from build123d import *

# Parameters (mm, degrees)
SKETCH1_W           = 38.1
SKETCH1_H           = 25.4
BOSS_EXTRUDE1_DEPTH = 90.1598
SKETCH2_W           = 25.4
SKETCH2_H           = 40.96
BOSS_EXTRUDE2_DEPTH = 30.0228
SKETCH3_W           = 25.4
SKETCH3_H           = 40.96
BOSS_EXTRUDE3_DEPTH = 30.0228
BOSS_EXTRUDE4_DEPTH = 110.0074
BOSS_EXTRUDE5_DEPTH = 110.0074
SKETCH8_R           = 3.81
CUT_EXTRUDE1_DEPTH  = 25.4


with BuildPart() as part:
    # Sketch1 → Boss-Extrude1 (new body)
    with BuildSketch(Plane(origin=(0, 0, 0), x_dir=(1, 0, 0), z_dir=(0, 1, 0))):
        with Locations((5.061883246, 0.142486096)):
            Rectangle(SKETCH1_W, SKETCH1_H)
    extrude(amount=BOSS_EXTRUDE1_DEPTH)

    # Sketch2 → Boss-Extrude2 (add)
    with BuildSketch(Plane(origin=(24.111883246, 0, 0), x_dir=(0, 0, -1), z_dir=(1, 0, 0))):
        with Locations((0.142486096, 69.6798)):
            Rectangle(SKETCH2_W, SKETCH2_H)
    extrude(amount=BOSS_EXTRUDE2_DEPTH)

    # Sketch3 → Boss-Extrude3 (add)
    with BuildSketch(Plane.ZY.offset(13.988116754)):
        with Locations((-0.142486096, 69.6798)):
            Rectangle(SKETCH3_W, SKETCH3_H)
    extrude(amount=BOSS_EXTRUDE3_DEPTH)

    # Sketch4 → Boss-Extrude4 (add)
    with BuildSketch(Plane(origin=(0, 0, -12.842486096), x_dir=(-1, 0, 0), z_dir=(0, 0, -1))):
        Polygon((-54.134683246, 90.1598), (-54.134683246, 49.1998), (-34.576683246, 49.1998), (-34.576683246, 70.6018), align=None)
    extrude(amount=BOSS_EXTRUDE4_DEPTH)

    # Sketch5 → Boss-Extrude5 (add)
    with BuildSketch(Plane(origin=(0, 0, -12.842486096), x_dir=(-1, 0, 0), z_dir=(0, 0, -1))):
        Polygon((44.010916754, 90.1598), (44.010916754, 49.1998), (24.452916754, 49.1998), (24.452916754, 70.6018), align=None)
    extrude(amount=BOSS_EXTRUDE5_DEPTH)

    # Sketch8 → Cut-Extrude1 (cut)
    with BuildSketch(Plane.XZ):
        with Locations(Location((-4.938116754, -0.142486096, 0), (0, 0, 270))):
            Circle(SKETCH8_R)
        with Locations(Location((15.061883246, -0.142486096, 0), (0, 0, 270))):
            Circle(SKETCH8_R)
    extrude(amount=-CUT_EXTRUDE1_DEPTH, mode=Mode.SUBTRACT)


solid = part.part
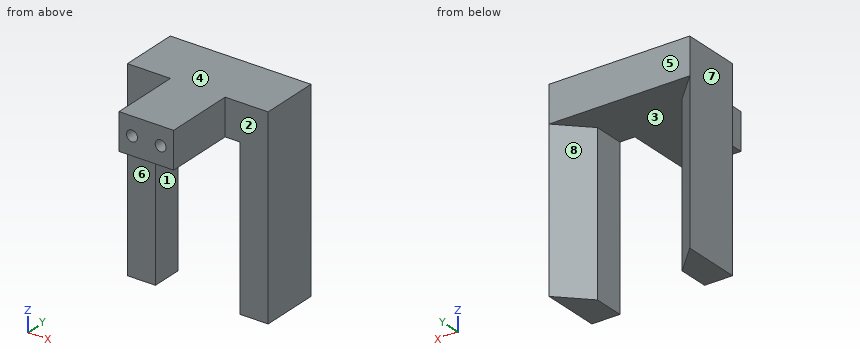
Source: CAD feature listing. Evaluate the final solid. Frame: model axes, mm. Face numbers are marked on the shaded views. A direction names the side the tool comes from. Give positions to 0.01 mm unless a question says otherwise; leave off trailing zeros. Write each loop counter-clockwise with the first axis right and the second up, starting at its lowest first coordinate (ties: lowest second). Pieces come first, ordered by that corner, then holes. Notation, with made-up numbers: M 34.25,58.25 L 77.25,58.25 A20 cw 77.25,84.25 Z; hole C 44,-31.5 d5. An arc over 180 degrees is marked long. Return JSON: item names as keys, results as strings. Group by question number.
1) Cut plane D-D, the plane x = -38. Output: boundary loops of the cut face in (y, z), plus the area to 3 significant figures.
2) Cut plane C-C, the plane y = 23. Output: boundary loops of the cut face in (x, z).
3) Cut plane A-A, the plane z = -76.5. Output: boundary loops of the cut face in (x, y), plus the area to 3 significant figures.
4) Material intervals for line 1 along X through (y, z) = (50, -93.5); line 2 along X through (y, z) = (43.5, -10); line 3 along Z through (x, y) = (-9.5, 44), sorted ascending. Write a range as [from, to].
5) Pin query (flat end, axial travel): P1, Ø1.5, axis at y = 23.5, z = -4.5, coming from the +X side; P2, Ø15, axis at x = 33, z = -29, coming from the -Y side; P3, Ø2.5, axis at x = -6.5, z = 1, coming from the -Y side. Return the tip coordinate at first contact, or that it passes through.
6) Cut plane B-B, the plane y = 64.5. Output: boundary loops of the cut face in (x, z), plus the area to 3 significant figures.
7) Set-up query: the marked faces 1, 2, 3, 4 and 5. Return all of +Z, -Z, +X, -X, +Y, -Y with unobstructed straight access to the full face (end or side cutting, diameter ignored); none if empty.
8) Pull-direction query (X, two-part tool) for the marked faces 6, 7 and 8; classes: pulls with the +X half, pulls with the -X half, needs draft (parallel to the pull), parting line crosses it, or undercut.
Recorded:
{
 "1": {"outline": "M 49.2,-122.85 L 84.15,-122.85 L 84.15,-12.84 L 90.16,-12.84 L 90.16,12.56 L 49.2,12.56 Z", "area": "4,890 mm²"},
 "2": {"outline": "M -13.99,-12.84 L 24.11,-12.84 L 24.11,12.56 L -13.99,12.56 Z; hole C -4.94,-0.14 d7.62; hole C 15.06,-0.14 d7.62"},
 "3": {"outline": "M -44.01,49.2 L -24.45,49.2 L -24.45,70.6 L -44.01,90.16 Z; M 34.58,49.2 L 54.13,49.2 L 54.13,90.16 L 34.58,70.6 Z", "area": "1,220 mm²"},
 "4": {"line 1": "x = [-44.01, -24.45], [34.58, 54.13]", "line 2": "x = [-13.99, 24.11]", "line 3": "z = [-12.84, 12.56]"},
 "5": {"P1": "stops at x = 24.11", "P2": "stops at y = 49.2", "P3": "stops at y = 25.4"},
 "6": {"outline": "M -44.01,-122.85 L -24.45,-122.85 L -24.45,-12.84 L 34.58,-12.84 L 34.58,-122.85 L 54.13,-122.85 L 54.13,12.56 L -44.01,12.56 Z", "area": "6,800 mm²"},
 "7": {"face 1": "-Z, +Y, -Y", "face 2": "+Z, -Z, +X, -Y", "face 3": "-Z, +Y", "face 4": "+Z, +X, -X, +Y, -Y", "face 5": "+Z, -Z, +X, -X, +Y"},
 "8": {"face 6": "needs draft", "face 7": "pulls with the -X half", "face 8": "undercut"}
}
